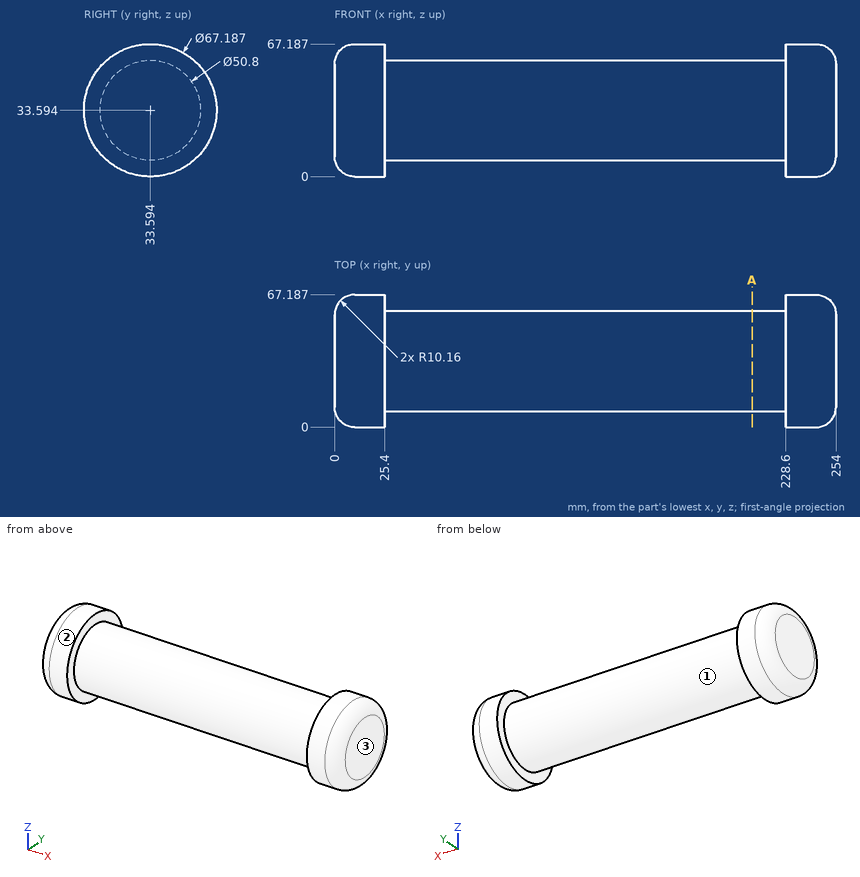
Design review of the part shown in the three views and the two pictorial views. Dimensions are in mm from the part's minimum x, y and z. Give positions to 0.01 mm unless a question says otherwise; leave off trailing zeros. Order: outer loops, then holes, each group sorted by start corner. A loop starts at its lowest first (then second) coordinate and runs counter-clockwise, first axis right, second up. Notation, with made-up numbers: (89, -22) -> (128, -22) arc R13 ccw to (128, 1) -> close; hole circle Ø9 at (34.25, 1). An arc over 180 degrees is marked (long way). Write each question's results on one line, items separated by ' | '. Start each with the question number.
Q1. For pin 1 (5 mm diameter, centred on x = 107.5, z = 29, fed in from +Y); pin 2 (8 mm diameter, centred on y = 10.5, z = 49, fed in from +X) (1 decimal); pin 3 (12 mm diameter, centred on x = 116, y = 50.5, fed in from -Z) (1 decimal), all flat-tipped, find the tip position at first contact; note any pin that passes through.
Q2. Wall thickness on L1, parallel to X at y = 8, z = 30.5 (1 decimal); L2, parallel to X at y = 9.5, z = 11.5; L3, parallel to Y at x = 180.5, z = 35 (1 decimal): over which ranges is each line inside the solid? List them lowest first. Write a range as from..to.
Q3. Add section A-A on x = 211.5. Give the boundary of the cut face in (y, z).
Q4. Mouldability with a two-part tool opening along X and no side actions: class the marked faces 1, 2 and 3 as +X half, -X half, draft (parallel to the pull), parting line (faces both ways), or undercut.
Found:
1) pin 1: stops at y = 58.91 | pin 2: stops at x = 254 | pin 3: stops at z = 10.7
2) L1: x = 0.3..25.4, 228.6..253.7 | L2: x = 5.97..25.4, 228.6..248.03 | L3: y = 8.2..59
3) outline: circle Ø50.8 at (33.59, 33.59)
4) face 1: undercut | face 2: draft | face 3: +X half
